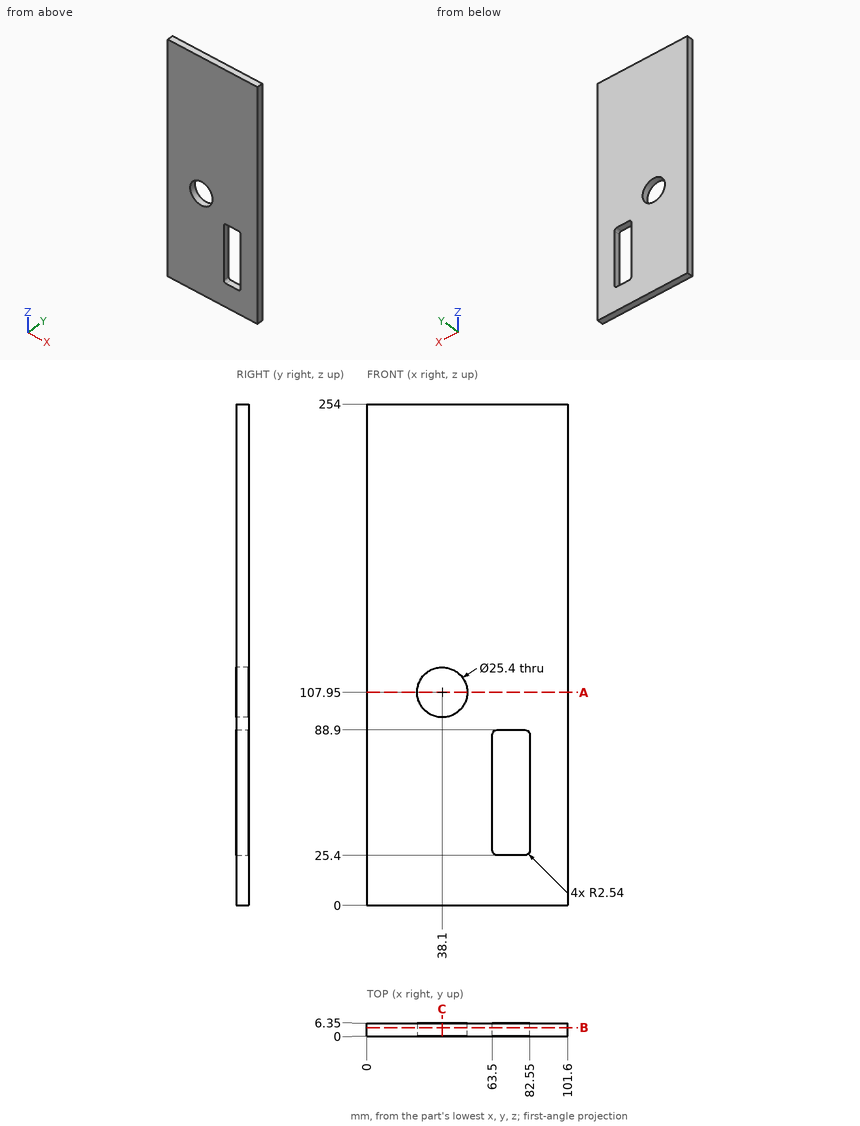
Check sheet for the drawn part. Datum: minimum x, y, z corner. Units: mm. Give positions to 0.01 mm unless a question says otherwise; leave off trailing zeros. Order: outer loops, then holes, each group sorted by start corner. A loop starts at its lowest first (then second) coordinate and runs counter-clockwise, first axis right, second up. Notation, with made-up numbers: (-33, -15.5) - (0, -15.5) arc R32 cw to (0, 19.5) - close; hole circle Ø8 at (55.25, 34.5). An arc over 180 degrees is marked (long way). Answer as a JSON object with one key per item and string values.
(1) Cross-section at B-B (y = 4.25). Record the cut outline in (x, z).
Report:
{"outline": "(0, 0) - (101.6, 0) - (101.6, 254) - (0, 254) - close; hole circle Ø25.4 at (38.1, 107.95); hole (63.5, 27.94) arc R2.54 ccw to (66.04, 25.4) - (80.01, 25.4) arc R2.54 ccw to (82.55, 27.94) - (82.55, 86.36) arc R2.54 ccw to (80.01, 88.9) - (66.04, 88.9) arc R2.54 ccw to (63.5, 86.36) - close"}
(2) Material ranges on line 1 (X direction, y = 2.5, z = 45); line 2 (Z direction, x = 38.1, y = 3); line 3 (X direction, y = 2, z = 107.95), recorded low to high.
Report:
{"line 1": "0 to 63.5, 82.55 to 101.6", "line 2": "0 to 95.25, 120.65 to 254", "line 3": "0 to 25.4, 50.8 to 101.6"}
(3) Cross-section at C-C (x = 38.1). Record the cut outline in (y, z).
Report:
{"outline": "(0, 0) - (6.35, 0) - (6.35, 95.25) - (0, 95.25) - close; (0, 120.65) - (6.35, 120.65) - (6.35, 254) - (0, 254) - close"}
(4) Depth check by flat-ended pin: pin 1 Ø1.9 at (x, y) = (76.5, 2) entering from -Z; pin 2 Ø10 at (x, z) = (34.5, 102) entering from +Y. Enter the tip coordinate at first touch or a pass-through.
Report:
{"pin 1": "z = 0", "pin 2": "through"}
(5) Cross-section at A-A (z = 107.95). Record the cut outline in (x, y), then the cut area to 3 significant figures.
Report:
{"outline": "(0, 0) - (25.4, 0) - (25.4, 6.35) - (0, 6.35) - close; (50.8, 0) - (101.6, 0) - (101.6, 6.35) - (50.8, 6.35) - close", "area": "484 mm^2"}
